Design review of the part built by this model. Coordinates are the model's own, in mm. A direction names the side the tool comes from. Round coordinates to 2 decimals unless told otherwise and drop trailing zeros. Order: outer loops, then holes, each group sorted by start corner. A loop starts at its lowest first (then second) coordinate and runs counter-clockwise, first axis right, second up. Notation, with made-up numbers: (85, -35) - (98, -35) arc R13 cw to (98, -11) - close; hole circle Ø1 at (7, 13). An arc over 180 degrees is marked (long way). Write item = value, one per line.
from build123d import *
from OCP.BRepFilletAPI import BRepFilletAPI_MakeChamfer

# Parameters (mm, degrees)
SKETCH1_R               = 2.375
BOSS_EXTRUDE1_DEPTH     = 0.55
SKETCH2_R               = 1.875
BOSS_EXTRUDE2_DEPTH     = 1.7
SKETCH3_R               = 2.5
BOSS_EXTRUDE3_DEPTH     = 2
SKETCH4_R               = 2.25
BOSS_EXTRUDE4_DEPTH     = 0.8
CUT_EXTRUDE1_REACH      = 8.165
SKETCH5_W               = 0.75
SKETCH5_H               = 6.07376998
CHAMFER1_SIZE           = 0.4
CHAMFER1_SIZE2          = 0.692820323
SKETCH6_W               = 6.999273813
SKETCH6_H               = 5.334981493
SKETCH6_W_2             = 6.558585844
SKETCH6_H_2             = 3.75
CUT_EXTRUDE3_DEPTH      = 2
FILLET2_R               = 1
SKETCH7_R               = 1
CUT_EXTRUDE4_DEPTH      = 2
CUT_EXTRUDE5_DEPTH      = 3
CUT_EXTRUDE5_DEPTH_BACK = 10
SKETCH9_W               = 3.309409713
SKETCH9_H               = 2.920914296
FILLET3_R               = 1.5


with BuildPart() as part:
    # Sketch1 → Boss-Extrude1 (new body)
    with BuildSketch(Plane.XY):
        Circle(SKETCH1_R)
    extrude(amount=BOSS_EXTRUDE1_DEPTH)

    # Sketch2 → Boss-Extrude2 (add)
    with BuildSketch(Plane.XY.offset(0.55)):
        Circle(SKETCH2_R)
    extrude(amount=BOSS_EXTRUDE2_DEPTH)

    # Sketch3 → Boss-Extrude3 (add)
    with BuildSketch(Plane(origin=(0, 0, 0), x_dir=(-1, 0, 0), z_dir=(0, 0, -1))):
        Circle(SKETCH3_R)
    extrude(amount=BOSS_EXTRUDE3_DEPTH)

    # Sketch4 → Boss-Extrude4 (add)
    with BuildSketch(Plane.XY.offset(2.25)):
        Circle(SKETCH4_R)
    extrude(amount=BOSS_EXTRUDE4_DEPTH)

    # Cut-Extrude1: up to this face of the body (flat: up to its plane)
    cut_extrude1_end = Plane(part.part.faces().sort_by_distance((-2.307824856, 0, 0.55))[0])
    # Sketch5 → Cut-Extrude1 (cut, up to the picked face)
    with BuildSketch(Plane.XY.offset(3.05), mode=Mode.PRIVATE) as cut_extrude1_sk1:
        Rectangle(SKETCH5_W, SKETCH5_H)
    cut_extrude1_tool1 = split(extrude(cut_extrude1_sk1.sketch, amount=-CUT_EXTRUDE1_REACH, mode=Mode.PRIVATE), bisect_by=cut_extrude1_end, keep=Keep.BOTH, mode=Mode.PRIVATE)
    add(cut_extrude1_tool1.solids().sort_by(Axis((0, 0, 3.05), (0, 0, -1)))[0], mode=Mode.SUBTRACT)

    # Chamfer1: one chamfer whose edges measure the first distance from different faces: ONE call of the kernel's chamfer builder (chamfer() names one face for all edges)
    chamfer1_edges_1 = [part.edges().sort_by_distance(p)[0] for p in [
        (-2.25, 0, 3.05),
    ]]
    chamfer1_side_1 = [part.faces().sort_by_distance(p)[0] for p in [
        (-2.25, 0, 2.65),
    ]]
    chamfer1_edges_2 = [part.edges().sort_by_distance(p)[0] for p in [
        (2.25, 0, 3.05),
    ]]
    chamfer1_side_2 = [part.faces().sort_by_distance(p)[0] for p in [
        (2.25, 0, 2.65),
    ]]
    chamfer1 = BRepFilletAPI_MakeChamfer(part.part.solid().wrapped)
    for e in chamfer1_edges_1:
        chamfer1.Add(CHAMFER1_SIZE, CHAMFER1_SIZE2, e.wrapped, chamfer1_side_1[0].wrapped)  # the first distance lies on this face
    for e in chamfer1_edges_2:
        chamfer1.Add(CHAMFER1_SIZE, CHAMFER1_SIZE2, e.wrapped, chamfer1_side_2[0].wrapped)  # the first distance lies on this face
    add(Compound.cast(chamfer1.Shape()), mode=Mode.REPLACE)

    # Sketch6 → Cut-Extrude3 (cut)
    with BuildSketch(Plane.XY.offset(3.05)):
        with Locations((0.047792, -0.043471688)):
            Rectangle(SKETCH6_W, SKETCH6_H)
        Rectangle(SKETCH6_W_2, SKETCH6_H_2, mode=Mode.SUBTRACT)
    extrude(amount=-CUT_EXTRUDE3_DEPTH, mode=Mode.SUBTRACT)

    # Fillet2
    fillet2_edges = [part.edges().sort_by_distance(p)[0] for p in [
        (-1.243734296, 1.875, 2.45),
        (1.243734296, 1.875, 2.45),
        (-1.243734296, -1.875, 2.45),
        (1.243734296, -1.875, 2.45),
    ]]
    fillet(fillet2_edges, radius=FILLET2_R)

    # Sketch7 → Cut-Extrude4 (cut)
    with BuildSketch(Plane(origin=(0, 0, -2), x_dir=(-1, 0, 0), z_dir=(0, 0, -1))):
        Circle(SKETCH7_R)
    extrude(amount=-CUT_EXTRUDE4_DEPTH, mode=Mode.SUBTRACT)

    # Sketch9 → Cut-Extrude5 (cut, two sides: drawn at the far end of the back side and taken through both)
    with BuildSketch(Plane(origin=(0, 0, 0), x_dir=(1, 0, 0), z_dir=(0, 1, 0)).offset(-CUT_EXTRUDE5_DEPTH_BACK)):
        with Locations((1.654704857, -2.010457148)):
            Rectangle(SKETCH9_W, SKETCH9_H)
    extrude(amount=CUT_EXTRUDE5_DEPTH + CUT_EXTRUDE5_DEPTH_BACK, mode=Mode.SUBTRACT)

    # Fillet3
    fillet3_edges = [part.edges().sort_by_distance(p)[0] for p in [
        (-0.375, 0, 0.55),
    ]]
    fillet(fillet3_edges, radius=FILLET3_R)


solid = part.part
1) To check wall thickness, follow L1, parallel to Y at x = 0, z = -0.45; L2, parallel to X at y = 0.05, z = 0.1; L3, parallel to Z at x = 2.05, y = 0.65. State the ranges of each line that lie inside material, in increasing order. Write a range as from..to.
Findings:
L1 = -2.5..-1, 1..2.5
L2 = -2.37..2.37
L3 = -2..0.55
2) We need section D-D on z = 2.4. Write out the cut boundary in (x, y) (3 decimals).
Findings:
outline = (-1.607, -1.575) arc R1 ccw to (-0.893, -1.875) - (-0.375, -1.875) - (-0.375, 1.875) - (-0.893, 1.875) arc R1 ccw to (-1.607, 1.575) arc R2.25 ccw to start
3) For faces 4 (the cylindrical face through (0, -1, -1)), 5 (the flat face through (-2.01, 0.29, 2.25)), 6 (the flat face through (-1, 0, 3.05)), 7 (the flat face through (-0.375, 0, 2.6)), list the 3-axis set-ups (+Z, -Z, +X, -X, +Y, -Y) from which the entire face can be reached by the end or side of a thin tool; tool diameter is ignored.
Findings:
face_4 = -Z
face_5 = -X
face_6 = +Z, +X, -X, +Y, -Y
face_7 = +Z, +X, +Y, -Y
4) We need section B-B on z = -0.15. Write out the cut boundary in (x, y), and give its area (3 significant figures).
Findings:
outline = circle Ø5 at (0, 0); hole circle Ø2 at (0, 0)
area = 16.5 mm^2
5) The part is to be moulded in two halves that separate along Y. For faces 1 (the flat face through (2, 0, 0.55)), 2 (the cylindrical face through (1.096, -2.107, 0.271)), 3 (the flat face through (0, 0, 0)), say which applies: released by +Y, released by -Y, zero draft, split by the parting line, or undercut.
Findings:
face_1 = zero draft
face_2 = split by the parting line
face_3 = undercut
6) Clearance check with flat-ended pins moving along their axes: pin 1 Ø1.6 at (x, y) = (0, 0) entering from -Z; pin 2 Ø1.5 at (x, z) = (-1, 1) entering from +Y; pin 3 Ø0.5 at (y, z) = (-0.5, 2.5) entering from +X (3 decimals). State where each tip first meets the part, or that it passes through.
Findings:
pin_1 = 0
pin_2 = 2.34
pin_3 = -0.375
7) We need section A-A on y = 0. Write out the cut boundary in (x, z) (3 decimals), and give its area (3 significant figures).
Findings:
outline = (-2.5, -2) - (-1, -2) - (-1, 0) - (1, 0) - (1, -2) - (2.5, -2) - (2.5, 0) - (2.375, 0) - (2.375, 0.55) - (1.125, 0.55) arc R1.5 cw to (-0.375, 2.05) - (-0.375, 3.05) - (-1.557, 3.05) - (-2.25, 2.65) - (-2.25, 2.25) - (-1.875, 2.25) - (-1.875, 0.55) - (-2.375, 0.55) - (-2.375, 0) - (-2.5, 0) - close
area = 13.0 mm^2
